Input: part model. Units: mm. Frame: model coordinates. Face numbers are marked on the shaded views. A direction names the side the tool comes from. Give positions to 0.01 mm unless a question says otherwise; leave off trailing zeros. Write each loop counter-clockwise with the first axis right and the second up, starting at its lowest first coordinate (ties: lowest second). Pieces come first, ordered by that corner, then holes.
```python
from build123d import *

# Parameters (mm, degrees)
BOSS_EXTRUDE1_DEPTH = 1.27
BOSS_EXTRUDE2_DEPTH = 2.03


with BuildPart() as part:
    # Sketch1 → Revolve1 (revolve)
    with BuildSketch(Plane(origin=(0, 0, 0), x_dir=(1, 0, 0), z_dir=(0, 1, 0))):
        Polygon((0, 0), (2.1, 0), (2.1, 3), (4.165, 4.73), (4.3, 24.44), (5.33, 24.44), (5.33, 27.1), (6.45, 27.1), (6.45, 28.62), (0, 28.62), align=None)
    revolve(axis=Axis((0, 0, -28.62), (0, 0, 1)))

    # Sketch2 → Boss-Extrude1 (add)
    with BuildSketch(Plane(origin=(0, 0, -28.62), x_dir=(-1, 0, 0), z_dir=(0, 0, -1))):
        with BuildLine():
            Line((5.206517503, 3.83254491), (2.416017403, 7.623443114))
            ThreePointArc((2.416017403, 7.623443114), (0, 8.845), (-2.416017403, 7.623443114))
            Line((-2.416017403, 7.623443114), (-5.206517503, 3.83254491))
            ThreePointArc((-5.206517503, 3.83254491), (0, -6.465), (5.206517503, 3.83254491))
        make_face()
    extrude(amount=BOSS_EXTRUDE1_DEPTH)

    # Sketch3 → Boss-Extrude2 (add, symmetric)
    with BuildSketch(Plane(origin=(0, 0, 0), x_dir=(0, 0, -1), z_dir=(1, 0, 0))):
        with BuildLine():
            Line((29.89, -5.667887402), (29.89, -9.59312184))
            ThreePointArc((29.89, -9.59312184), (29.385325952, -10.18), (28.729482517, -9.768914535))
            Line((28.729482517, -9.768914535), (27.803917735, -5.667887402))
            Line((27.803917735, -5.667887402), (29.89, -5.667887402))
        make_face()
    extrude(amount=BOSS_EXTRUDE2_DEPTH, both=True)


solid = part.part
```
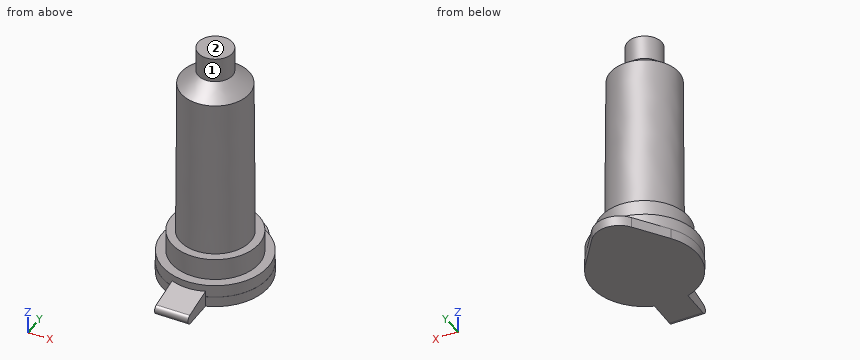
Q1. Section C-C, the plane z = -23.75. Return the cut outline in (x, y).
Q2. Material intervals for line 1 along Z through (x, y) = (1.5, 5.5); line 2 along Z through (x, y) = (-2.5, 4); line 3 along Y through (x, z) = (1.5, -9.25), sorted ascending.
Q3. Pin query (flat end, axial travel): pin 1 (4 mm diameter, centred on x = -0.5, y = -0.5, fed in from +Z); pin 2 (2 mm diameter, centred on y = -8, z = -28.5, fed in from +X); pin 3 (4 mm diameter, centred on x = -5, y = 4.5, fed in from +Z); pin 4 (1 mm diameter, centred on y = -8.5, z = -29, fed in from -X). Return the tip coordinate at first contact, or that it passes through.
Q4. Access query for the marked faces 1 and 2. Directions: +Z, -Z, +X, -X, +Y, -Y. A direction counts if a zero-diameter tool reaches every point of the face in a straight line with its end or side. Return the directions, or none.
Q5. Section A-A, the plane z = -2. Return the cut outline in (x, y), then the cut area to 3 significant figures.
Q6. Section B-B, the plane y = -7. Return the cut outline in (x, z), then the cut area to 3 significant figures.
Solutions:
1. outline: circle Ø8.59 at (0, 0)
2. line 1: z = -29.89 to -27.1
2. line 2: z = -29.89 to -24.44
2. line 3: y = -3.92 to 3.92
3. pin 1: stops at z = 0
3. pin 2: stops at x = 2.03
3. pin 3: stops at z = -24.44
3. pin 4: stops at x = -2.03
4. face 1: +Z
4. face 2: +Z, +X, -X, +Y, -Y
5. outline: circle Ø4.2 at (0, 0)
5. area: 13.9 mm2
6. outline: (-2.03, -29.89) - (2.03, -29.89) - (2.03, -28.1) - (-2.03, -28.1) - close
6. area: 7.25 mm2
